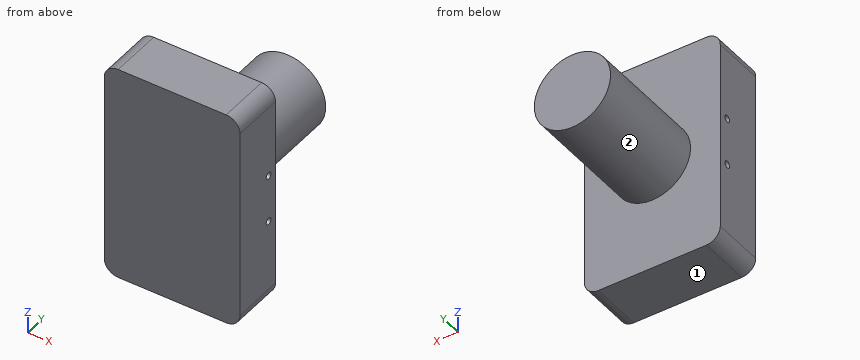
Autodesk Inventor part; units mm, degrees
ref_plane "YZ Plane" through (0, 0, 0) normal (1, 0, 0) x (0, 1, 0)
ref_plane "XZ Plane" through (0, 0, 0) normal (0, 1, 0) x (-1, 0, 0)
ref_plane "XY Plane" through (0, 0, 0) normal (0, 0, 1) x (1, 0, 0)
sketch "Sketch1" plane through (0, 0, 0) normal (0, 1, 0) x (-1, 0, 0)
  line L0 (0, 0) -> (58.75, 0)
  line L1 (58.75, 0) -> (58.75, -94.75)
  line L2 (58.75, -94.75) -> (0, -94.75)
  line L3 (0, -94.75) -> (0, 0)
  dimension "d0" = 58.75
  dimension "d1" = 94.75
extrude "Extrusion1" add sketch "Sketch1" along normal blind 22.6
sketch "Sketch2" plane through (0, 22.6, 0) normal (0, 1, 0) x (1, 0, 0)
  line L0 (-58.75, 0) -> (0, 0)
  line L1 (-29.375, 0) -> (-29.375, 94.75)
  line L2 (0, 94.75) -> (-58.75, 94.75)
  line L3 (-58.75, 94.75) -> (-58.75, 0)
  line L4 (-58.75, 47.375) -> (0, 47.375)
  line L5 (0, 0) -> (0, 94.75)
  circle A0 centre (-29.375, 47.375) radius 16.5
  dimension "d4" = 33
extrude "Extrusion2" add sketch "Sketch2" along normal blind 51 contours A0 L4 L1 | L1 L4 A0 | A0 L1 L4 | L1 A0 L4
fillet "Fillet1" radius 6 4 edges at (0, 11.3, 0) (0, 11.3, -94.75) (-58.75, 11.3, 0) (-58.75, 11.3, -94.75)
sketch "Sketch3" plane through (-58.75, 0, -88.75) normal (-1, 0, 0) x (0, 0, 1)
  line L0 (82.75, 22.6) -> (88.75, 22.6)
  line L1 (88.75, 22.6) -> (51.75, 22.6)
  line L2 (24.875, 22.6) -> (57.875, 22.6)
  line L3 (51.75, 22.6) -> (51.75, 18.2)
  circle A0 centre (51.75, 18.2) radius 1.5
  line L4 (41.375, 22.6) -> (41.375, 4.2655)
  circle A1 centre (31, 18.2) radius 1.5
  point P0 (88.75, 0)
  dimension "d8" = 37
  dimension "d9" = 4.4
  dimension "d10" = 3
extrude "Extrusion3" cut sketch "Sketch3" against normal blind 70
properties part number "camera_v2"
Read the model definition and answer for the solid it produces. Units are mm, in the model's axes. Face numbers are marked on the shaded views. A direction names the side the tool comes from. Coordinates: 2 decimals unless noted, no trailing zeros. Loops run counter-clockwise (first coordinate to the right, second up) from the corner with the lowest first, then second, coordinate; pieces in that order, holes last. Notation, with made-up numbers: (44.5, -6) -> (84.5, -6) arc R10 ccw to (84.5, 8) -> close; hole circle Ø4 at (13, 80). An arc over 180 degrees is marked (long way). Answer in a Markdown table with one row per item.
Item 1: Each of these flat-tipped pins is pushed along its axis until it touches: P1, Ø2.5, axis at y = 18.2, z = -37, coming from the -X side; P2, Ø12, axis at x = -44.5, y = 38.5, coming from the +Z side; P3, Ø8, axis at x = -21, z = -67, coming from the +Y side; P4, Ø1, axis at x = -21, y = 57, coming from the -Z side. Where does it stop, or does it pass through?
Returned:
| item | result |
|---|---|
| P1 | passes through |
| P2 | stops at z = -33.63 |
| P3 | stops at y = 22.6 |
| P4 | stops at z = -61.87 |
Item 2: A cutting plane is placed at C-C on z = -37. Determine the outline of the cut face in (x, y), plus the area to 3 significant figures.
Returned:
| item | result |
|---|---|
| outline | (-58.75, 0) -> (0, 0) -> (0, 16.7) -> (-58.75, 16.7) -> close; (-58.75, 19.7) -> (0, 19.7) -> (0, 22.6) -> (-16.54, 22.6) -> (-16.54, 73.6) -> (-42.21, 73.6) -> (-42.21, 22.6) -> (-58.75, 22.6) -> close |
| area | 2,460 mm^2 |
Item 3: A cutting plane is placed at D-D on x = -18. Determine the outline of the cut face in (y, z).
Returned:
| item | result |
|---|---|
| outline | (0, -94.75) -> (22.6, -94.75) -> (22.6, -59.33) -> (73.6, -59.33) -> (73.6, -35.42) -> (22.6, -35.42) -> (22.6, 0) -> (0, 0) -> close; hole circle Ø3 at (18.2, -57.75); hole circle Ø3 at (18.2, -37) |
Item 4: For the marked faces 1 and 2, determine the directions among +Z, -Z, +X, -X, +Y, -Y from which every point of the face is accessible in a straight line to the end or side of a thin tool.
Returned:
| item | result |
|---|---|
| face 1 | -Z, +X, -X, +Y, -Y |
| face 2 | +Y |
Item 5: Straight lines are drawn through the part: line 1 along Z through (x, y) = (-45, 18); line 2 along Y through (x, z) = (-28, -57.5); line 3 along Y through (x, z) = (-9, -72.5). For each, find the intervals that lie inside material, in ascending order. Write a range as [from, to].
Returned:
| item | result |
|---|---|
| line 1 | z = [-94.75, -59.24], [-56.26, -38.49], [-35.51, 0] |
| line 2 | y = [0, 16.72], [19.68, 73.6] |
| line 3 | y = [0, 22.6] |
Item 6: A cutting plane is placed at A-A on y = 18.2. Determine the outline of the cut face in (x, z), plus the area to 3 significant figures.
Returned:
| item | result |
|---|---|
| outline | (-58.75, -88.75) arc R6 ccw to (-52.75, -94.75) -> (-6, -94.75) arc R6 ccw to (0, -88.75) -> (0, -59.25) -> (-58.75, -59.25) -> close; (-58.75, -56.25) -> (0, -56.25) -> (0, -38.5) -> (-58.75, -38.5) -> close; (-58.75, -35.5) -> (0, -35.5) -> (0, -6) arc R6 ccw to (-6, 0) -> (-52.75, 0) arc R6 ccw to (-58.75, -6) -> close |
| area | 5,180 mm^2 |
Item 7: A cutting plane is placed at B-B on x = -25.5. Determine the outline of the cut face in (y, z), plus the area to 3 significant figures.
Returned:
| item | result |
|---|---|
| outline | (0, -94.75) -> (22.6, -94.75) -> (22.6, -63.41) -> (73.6, -63.41) -> (73.6, -31.34) -> (22.6, -31.34) -> (22.6, 0) -> (0, 0) -> close; hole circle Ø3 at (18.2, -57.75); hole circle Ø3 at (18.2, -37) |
| area | 3,760 mm^2 |
